```python
from build123d import *

# Parameters (mm, degrees)
SKETCH_1_W          = 148
SKETCH_1_H          = 200
SKETCH_1_R          = 2.5
EXTRUDE_1_DEPTH     = 2.5
SKETCH_2_R          = 2.5
CUT_EXTRUDE_1_DEPTH = 3


with BuildPart() as part:
    # 草图1 → 凸台-拉伸1 (new body)
    with BuildSketch(Plane.XY):
        Rectangle(SKETCH_1_W, SKETCH_1_H)
        with Locations((-58, -71.5)):
            Circle(SKETCH_1_R, mode=Mode.SUBTRACT)
        with Locations((-27.5, -71.5)):
            Circle(SKETCH_1_R, mode=Mode.SUBTRACT)
        with Locations((-42.75, -91)):
            Circle(SKETCH_1_R, mode=Mode.SUBTRACT)
        with Locations((42.75, -91)):
            Circle(SKETCH_1_R, mode=Mode.SUBTRACT)
        with Locations((58, -71.5)):
            Circle(SKETCH_1_R, mode=Mode.SUBTRACT)
        with Locations((27.5, -71.5)):
            Circle(SKETCH_1_R, mode=Mode.SUBTRACT)
    extrude(amount=EXTRUDE_1_DEPTH)

    # 草图2 → 切除-拉伸1 (cut)
    with BuildSketch(Plane.XY.offset(2.5)):
        with Locations((-56.5, -10)):
            Circle(SKETCH_2_R)
        with Locations((-24.5, -10)):
            Circle(SKETCH_2_R)
        with Locations((-56.5, 85)):
            Circle(SKETCH_2_R)
        with Locations((-24.5, 85)):
            Circle(SKETCH_2_R)
        with Locations((24.5, 85)):
            Circle(SKETCH_2_R)
        with Locations((56.5, 85)):
            Circle(SKETCH_2_R)
        with Locations((24.5, -10)):
            Circle(SKETCH_2_R)
        with Locations((56.5, -10)):
            Circle(SKETCH_2_R)
    extrude(amount=-CUT_EXTRUDE_1_DEPTH, mode=Mode.SUBTRACT)


solid = part.part
```
Geometry check sheet. Reference: the model listing, model coordinates, mm. Give positions to 0.01 mm unless a question says otherwise; leave off trailing zeros. Order: outer loops, then holes, each group sorted by start corner. A loop starts at its lowest first (then second) coordinate and runs counter-clockwise, first axis right, second up. Notation, with made-up numbers: (89.25, -3.5) - (111.25, -3.5) arc R22 ccw to (111.25, 15.5) - close; hole circle Ø1 at (-7, 75.5). An arc over 180 degrees is marked (long way). Write item = value, one per line. Start each with the question number.
1) Draft check along Y on faces 1 (the flat face through (-1, 1, 2.5)), 2 (the cylindrical face through (58.81, -10.96, 1.27)). Enter one of: released by +Y, released by -Y, zero draft, split by the parting line, or undercut.
2) Scan lines: L1, parallel to Y at x = 24.5, z = 1.4; L2, parallel to Y at x = -57, z = 1.3; L3, parallel to Y at x = 58.5, z = 0.5. Record each from-to range of solid material in increasing order.
3) Section check A-A (y = -71.5). Enter the section's corners in (x, z).
Geometry check:
q1.face_1 = zero draft
q1.face_2 = undercut
q2.L1 = -100 to -12.5, -7.5 to 82.5, 87.5 to 100
q2.L2 = -100 to -73.79, -69.21 to -12.45, -7.55 to 82.55, 87.45 to 100
q2.L3 = -100 to -73.95, -69.05 to -11.5, -8.5 to 83.5, 86.5 to 100
q3.outline = (-74, 0) - (-60.5, 0) - (-60.5, 2.5) - (-74, 2.5) - close; (-55.5, 0) - (-30, 0) - (-30, 2.5) - (-55.5, 2.5) - close; (-25, 0) - (25, 0) - (25, 2.5) - (-25, 2.5) - close; (30, 0) - (55.5, 0) - (55.5, 2.5) - (30, 2.5) - close; (60.5, 0) - (74, 0) - (74, 2.5) - (60.5, 2.5) - close
